Geometry: final body of the model. Coordinates: model frame, mm. A direction names the side the tool comes from. Coordinates: 2 decimals unless noted, no trailing zeros. Order: outer loops, then holes, each group sorted by start corner. A loop starts at its lowest first (then second) coordinate and runs counter-clockwise, first axis right, second up. Notation, with made-up numbers: (69, 12.5) -> (95, 12.5) arc R28 ccw to (95, 41.5) -> close; hole circle Ø8 at (50, -0.5). An arc over 180 degrees is marked (long way). Use one line per item in the form item = value.
```python
from build123d import *

# Parameters (mm, degrees)
SKETCH1_W           = 25
SKETCH1_H           = 25
SKETCH1_R           = 1.55
BOSS_EXTRUDE1_DEPTH = 3
SKETCH2_W           = 10.5
SKETCH2_H           = 18
CUT_EXTRUDE1_DEPTH  = 18.930421077
CUT_EXTRUDE2_DEPTH  = 18.930421077
FILLET2_R           = 3


with BuildPart() as part:
    # Sketch1 → Boss-Extrude1 (new body)
    with BuildSketch(Plane(origin=(0, 0, 0), x_dir=(1, 0, 0), z_dir=(0, 1, 0))):
        Rectangle(SKETCH1_W, SKETCH1_H)
        with Locations(Location((-9.5, 9.5, 0), (0, 0, 270))):
            Circle(SKETCH1_R, mode=Mode.SUBTRACT)
        with Locations(Location((-9.5, -9.5, 0), (0, 0, 270))):
            Circle(SKETCH1_R, mode=Mode.SUBTRACT)
    extrude(amount=-BOSS_EXTRUDE1_DEPTH)

    # Sketch2 → Cut-Extrude1 (cut, through all)
    with BuildSketch(Plane(origin=(0, 0, 0), x_dir=(1, 0, 0), z_dir=(0, 1, 0))):
        with Locations((7.25, -3.5)):
            Rectangle(SKETCH2_W, SKETCH2_H)
    extrude(amount=-CUT_EXTRUDE1_DEPTH, mode=Mode.SUBTRACT)

    # Sketch3 → Cut-Extrude2 (cut, through all)
    with BuildSketch(Plane(origin=(0, 0, 0), x_dir=(1, 0, 0), z_dir=(0, 1, 0))):
        with BuildLine():
            Line((-12.5, -12.5), (12.5, -12.5))
            Line((12.5, -12.5), (12.5, 12.5))
            ThreePointArc((12.5, 12.5), (5.17766953, -5.17766953), (-12.5, -12.5))
        make_face()
    extrude(amount=-CUT_EXTRUDE2_DEPTH, mode=Mode.SUBTRACT)

    # Fillet2
    fillet2_edges = [part.edges().sort_by_distance(p)[0] for p in [
        (-12.5, -1.5, 12.5),
        (-12.5, -1.5, -12.5),
        (12.5, -1.5, -12.5),
    ]]
    fillet(fillet2_edges, radius=FILLET2_R)


solid = part.part
```
1) Section C-C, the plane x = -3.5. Output: boundary loops of the cut face in (y, z).
Results found:
outline = (-3, -12.5) -> (0, -12.5) -> (0, 10.82) -> (-3, 10.82) -> close
2) Section A-A, the plane y = -1.6. Output: boundary loops of the cut face in (x, z).
Results found:
outline = (-12.5, -9.5) arc R3 ccw to (-9.5, -12.5) -> (9.29, -12.5) arc R3 ccw to (12.27, -9.09) arc R25 ccw to (11.5, -5.5) -> (2, -5.5) -> (2, 7.87) arc R25 ccw to (-9.09, 12.27) arc R3 ccw to (-12.5, 9.29) -> close; hole circle Ø3.1 at (-9.5, -9.5); hole circle Ø3.1 at (-9.5, 9.5)
3) Pull-direction query (Z, two-part tool) for faces 1 (the flat face through (-12.5, -1, 0)), 2 (the cylindrical face through (-10.44, -1.48, -10.73)), 3 (the cylindrical face through (11.955, -1.479, -7.307)); classes: released by +Z, released by -Z, zero draft, split by the parting line, or undercut.
Results found:
face_1 = zero draft
face_2 = undercut
face_3 = released by +Z
4) Access query for faces 4 (the flat face through (7, -1, -5.5)), 5 (the cylindrical face through (-11.013, -1.479, 9.164)). Directions: +Z, -Z, +X, -X, +Y, -Y. A direction counts if a zero-diameter tool reaches every point of the face in a straight line with its end or side. Return the directions, or none.
Results found:
face_4 = +Z, +X, +Y, -Y
face_5 = +Y, -Y
5) Section B-B, the plane z = -0.5. Output: boundary loops of the cut face in (x, y), and give its area (3 significant figures).
Results found:
outline = (-12.5, -3) -> (2, -3) -> (2, 0) -> (-12.5, 0) -> close
area = 43.5 mm2
6) Material intervals for probe 1 along X at (y, z) = (-0.8, -9.5); probe 2 along X at (y, z) = (-2, 9.5); probe 3 along X at (y, z) = (-0.4, 2.5), sorted ascending. Write a range as from..to.
Results found:
probe_1 = -12.5..-11.05, -7.95..12.29
probe_2 = -12.49..-11.05, -7.95..-0.63
probe_3 = -12.5..2
7) Contact query for flat-ended pins moving along their axis: P1, Ø1.5, axis at y = -1, z = 6.5, coming from the +X side; P2, Ø3, axis at x = -9.5, z = 9.5, coming from the +Y side; P3, Ø0.9, axis at x = 9, y = -2, coming from the +Z side. Output: stop coordinate, or through.
Results found:
P1 = 2
P2 = through
P3 = -5.5
